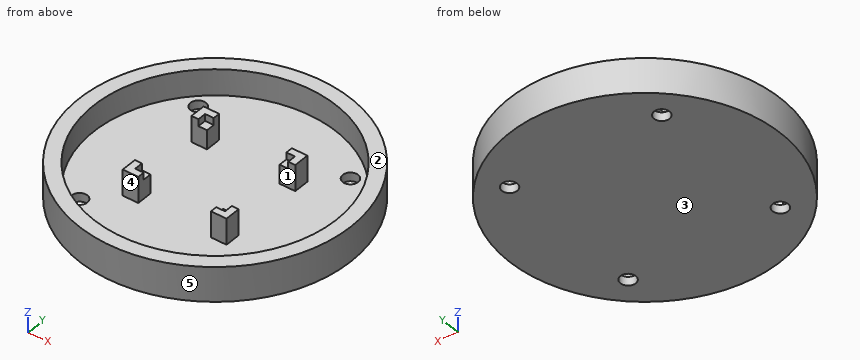
from build123d import *

# Parameters (mm, degrees)
SKETCH006_R     = 39.229987
PAD001_DEPTH    = 10
SKETCH007_R     = 35.030743
POCKET003_DEPTH = 7.5
SKETCH008_R     = 2.223377
SKETCH008_R_2   = 2.22785
SKETCH008_R_3   = 2.236068
POCKET004_DEPTH = 5
SKETCH011_W     = 4.5
SKETCH011_H     = 4.5
PAD002_DEPTH    = 7.5
SKETCH012_W     = 2.831394
SKETCH012_H     = 3.088426
POCKET005_DEPTH = 2
SKETCH013_W     = 2.956726
SKETCH013_H     = 2.855928
POCKET006_DEPTH = 2
SKETCH014_W     = 2.736649
SKETCH014_H     = 2.756396
POCKET007_DEPTH = 2
SKETCH015_W     = 2.695849
SKETCH015_H     = 2.640832
POCKET008_DEPTH = 2


with BuildPart() as part:
    # Sketch006 → Pad001 (new body)
    with BuildSketch(Plane.XY.offset(-10)):
        Circle(SKETCH006_R)
    extrude(amount=PAD001_DEPTH)

    # Sketch007 → Pocket003 (cut)
    with BuildSketch(Plane.XY):
        Circle(SKETCH007_R)
    extrude(amount=-POCKET003_DEPTH, mode=Mode.SUBTRACT)

    # Sketch008 → Pocket004 (cut)
    with BuildSketch(Plane.XY.offset(-7.5)):
        with Locations((22, -22)):
            Circle(SKETCH008_R)
        with Locations((22, 22)):
            Circle(SKETCH008_R_2)
        with Locations((-22, 22)):
            Circle(SKETCH008_R_3)
        with Locations((-22, -22)):
            Circle(SKETCH008_R_3)
    extrude(amount=-POCKET004_DEPTH, mode=Mode.SUBTRACT)

    # Sketch011 → Pad002 (new body)
    with BuildSketch(Plane.XY.offset(-7.5)):
        with Locations((12.75, 12.75)):
            Rectangle(SKETCH011_W, SKETCH011_H)
        with Locations((12.75, -12.75)):
            Rectangle(SKETCH011_W, SKETCH011_H)
        with Locations((-12.75, -12.75)):
            Rectangle(SKETCH011_W, SKETCH011_H)
        with Locations((-12.75, 12.75)):
            Rectangle(SKETCH011_W, SKETCH011_H)
    extrude(amount=PAD002_DEPTH)

    # Sketch012 → Pocket005 (cut)
    with BuildSketch(Plane.XY):
        with Locations((-11.575037, 11.434175)):
            Rectangle(SKETCH012_W, SKETCH012_H)
    extrude(amount=-POCKET005_DEPTH, mode=Mode.SUBTRACT)

    # Sketch013 → Pocket006 (cut)
    with BuildSketch(Plane.XY):
        with Locations((11.494347, 11.570308)):
            Rectangle(SKETCH013_W, SKETCH013_H)
    extrude(amount=-POCKET006_DEPTH, mode=Mode.SUBTRACT)

    # Sketch014 → Pocket007 (cut)
    with BuildSketch(Plane.XY):
        with Locations((11.6727, -11.659363)):
            Rectangle(SKETCH014_W, SKETCH014_H)
    extrude(amount=-POCKET007_DEPTH, mode=Mode.SUBTRACT)

    # Sketch015 → Pocket008 (cut)
    with BuildSketch(Plane.XY):
        with Locations((-11.611325, -11.666073)):
            Rectangle(SKETCH015_W, SKETCH015_H)
    extrude(amount=-POCKET008_DEPTH, mode=Mode.SUBTRACT)


solid = part.part
Read the model definition and answer for the solid it produces. Units are mm, in the model's axes. Face numbers are marked on the shaded views. A direction names the side the tool comes from. Round coordinates to 2 decimals unless told otherwise and drop trailing zeros. Loops run counter-clockwise (first coordinate to the right, second up) from the corner with the lowest first, then second, coordinate; pieces in that order, holes last.
Q1. Section B-B on y = 0 is taken. Write down the section's boundary in (x, z), and give its area (3 significant figures).
Q2. Section A-A on z = -6.5 is taken. Write down the section's boundary in (x, y), and give its area (3 significant figures).
Q3. Consider probe 1 along Y at (x, z) = (0, -4.25); probe 2 along Y at (x, z) = (-22, -9); probe 3 along Y at (x, z) = (-22.5, -9.25). Determine where each line is inside the solid, lowest interval first.
Q4. Determine the mould class of the marked faces 3, 4 and 5 for opening direction X: released by +X, released by -X, zero draft, split by the parting line, or undercut.
Q5. Each of these flat-tipped pins is pushed along its axis until it touches: pin 1 (2 mm diameter, centred on y = -24, z = -2, fed in from +X); pin 2 (5 mm diameter, centred on y = -12.5, z = -5, fed in from -X); pin 3 (1.5 mm diameter, centred on x = 8, z = -7, fed in from -Y); pin 4 (3.5 mm diameter, centred on x = -22, y = -22, fed in from +Z). Where does it stop, or does it pass through?
Q6. Which of the six approach directions +Z, -Z, +X, -X, +Y, -Y give full straight-line access (tool end or side, diameter ignored) to the marked faces 1 and 2?
Q7. Section C-C on x = -22 is taken. Write down the section's boundary in (y, z), and give its area (3 significant figures).
Output:
1. outline: (-39.23, -10) - (39.23, -10) - (39.23, 0) - (35.03, 0) - (35.03, -7.5) - (-35.03, -7.5) - (-35.03, 0) - (-39.23, 0) - close
1. area: 259 mm2
2. outline: circle Ø78.46 at (0, 0); (-15, -15) - (-10.5, -15) - (-10.5, -10.5) - (-15, -10.5) - close; (-15, 10.5) - (-10.5, 10.5) - (-10.5, 15) - (-15, 15) - close; (10.5, -15) - (15, -15) - (15, -10.5) - (10.5, -10.5) - close; (10.5, 10.5) - (15, 10.5) - (15, 15) - (10.5, 15) - close; hole circle Ø70.06 at (0, 0)
2. area: 1,060 mm2
3. probe 1: y = -39.23 to -35.03, 35.03 to 39.23
3. probe 2: y = -32.48 to -24.24, -19.76 to 19.76, 24.24 to 32.48
3. probe 3: y = -32.14 to -24.18, -19.82 to 19.82, 24.18 to 32.14
4. face 3: zero draft
4. face 4: undercut
4. face 5: split by the parting line
5. pin 1: stops at x = 31.78
5. pin 2: stops at x = -37.93
5. pin 3: stops at y = -38.55
5. pin 4: passes through
6. face 1: +Z
6. face 2: +Z, +X, -X, +Y, -Y
7. outline: (-32.48, -10) - (-24.24, -10) - (-24.24, -7.5) - (-27.26, -7.5) - (-27.26, 0) - (-32.48, 0) - close; (-19.76, -10) - (19.76, -10) - (19.76, -7.5) - (-19.76, -7.5) - close; (24.24, -10) - (32.48, -10) - (32.48, 0) - (27.26, 0) - (27.26, -7.5) - (24.24, -7.5) - close
7. area: 218 mm2
